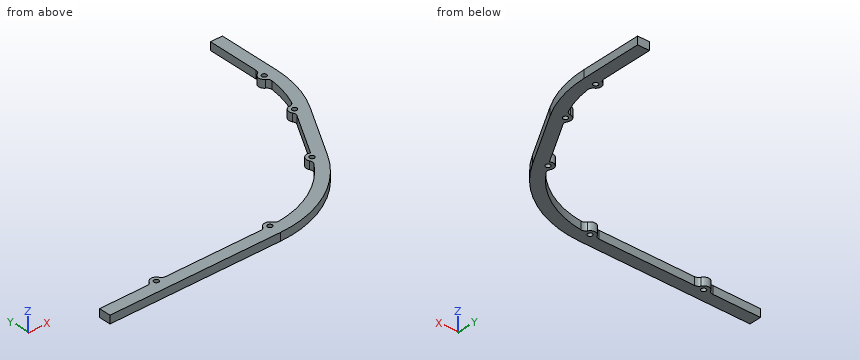
Solid Edge part; units mm, degrees
sketch "Sketch1" plane through (0.0007, 14.651, 5) normal (0, 0, 1) x (1, 0, 0)
  line L0 (-114.0407, 98.8093) -> (-57.2599, 131.5929)
  arc A0 (-54.1474, 131.5247) -> (-57.2599, 131.5929) centre (-55.7598, 128.9948) ccw
  arc A1 (-47.0142, 137.1861) -> (-48.7662, 134.4664) centre (-45.7662, 134.458) ccw
  arc A2 (-47.0142, 137.1861) -> (-26.9146, 142.5706) centre (-21.0226, 80.3698) cw
  arc A3 (-24.0376, 141.0909) -> (-26.9146, 142.5706) centre (-26.6317, 139.5839) ccw
  arc A4 (-15.245, 142.849) -> (-17.9063, 141.2336) centre (-15.245, 139.849) ccw
  line L1 (-15.245, 142.849) -> (15.2436, 142.849)
  arc A5 (17.905, 141.2336) -> (15.2436, 142.849) centre (15.2436, 139.849) ccw
  arc A6 (26.9132, 142.5696) -> (24.036, 141.0904) centre (26.6298, 139.583) ccw
  arc A7 (26.9132, 142.5696) -> (47.0027, 137.1869) centre (21.0099, 80.3561) cw
  arc A8 (48.7549, 134.4673) -> (47.0027, 137.1869) centre (45.7549, 134.4587) ccw
  arc A9 (57.2487, 131.5943) -> (54.1362, 131.526) centre (55.7487, 128.9962) ccw
  line L2 (57.2487, 131.5943) -> (114.0299, 98.8129)
  arc A10 (115.5271, 96.0833) -> (114.0299, 98.8129) centre (112.5299, 96.2148) ccw
  arc A11 (124.0003, 92.7805) -> (120.7849, 92.9052) centre (122.2944, 90.3127) ccw
  arc A12 (124.0003, 92.7805) -> (155.0355, 39.027) centre (82.7747, 33.1424) cw
  arc A13 (153.5358, 36.1799) -> (155.0355, 39.027) centre (152.0454, 38.7835) ccw
  arc A14 (155.2747, 27.3761) -> (153.6593, 30.0375) centre (152.2747, 27.3761) ccw
  line L3 (155.2747, 27.3761) -> (155.2747, -38.192)
  arc A15 (153.6593, -40.8534) -> (155.2747, -38.192) centre (152.2747, -38.192) ccw
  arc A16 (154.9954, -49.8615) -> (153.5161, -46.9844) centre (152.0088, -49.5782) ccw
  arc A17 (154.9954, -49.8615) -> (149.6134, -69.9554) centre (92.7533, -43.9583) cw
  arc A18 (146.8942, -71.7079) -> (149.6134, -69.9554) centre (146.8851, -68.7079) ccw
  arc A19 (144.0217, -80.2016) -> (143.9534, -77.0892) centre (141.4236, -78.7016) ccw
  line L4 (144.0217, -80.2016) -> (127.6444, -108.5679)
  arc A20 (122.7007, -116.5716) -> (122.8583, -113.3403) centre (120.256, -114.8329) ccw
  arc A21 (77.6703, -142.5696) -> (122.7007, -116.5716) centre (71.767, -80.3476) ccw
  arc A22 (74.7931, -141.0904) -> (77.6703, -142.5696) centre (77.3869, -139.583) ccw
  arc A23 (66.0007, -142.849) -> (68.6621, -141.2336) centre (66.0007, -139.849) ccw
  line L5 (5.7656, -142.849) -> (66.0007, -142.849)
  arc A24 (3.1042, -141.2336) -> (5.7656, -142.849) centre (5.7656, -139.849) ccw
  arc A25 (-5.767, -142.849) -> (-3.1056, -141.2336) centre (-5.767, -139.849) ccw
  line L6 (-66.0021, -142.849) -> (-5.767, -142.849)
  arc A26 (-68.6634, -141.2336) -> (-66.0021, -142.849) centre (-66.0021, -139.849) ccw
  arc A27 (-77.6716, -142.5694) -> (-74.7944, -141.0903) centre (-77.3881, -139.5828) ccw
  arc A28 (-122.6994, -116.5717) -> (-77.6716, -142.5694) centre (-71.7665, -80.349) ccw
  arc A29 (-122.857, -113.3404) -> (-122.6994, -116.5717) centre (-120.2547, -114.833) ccw
  arc A30 (-128.7762, -106.6053) -> (-126.0465, -108.1024) centre (-126.1781, -105.1053) ccw
  line L7 (-144.0218, -80.199) -> (-128.7762, -106.6053)
  arc A31 (-143.9535, -77.0865) -> (-144.0218, -80.199) centre (-141.4237, -78.699) ccw
  arc A32 (-149.6144, -69.9531) -> (-146.8949, -71.7053) centre (-146.8862, -68.7053) ccw
  arc A33 (-154.9987, -49.8585) -> (-149.6144, -69.9531) centre (-92.7672, -43.9523) ccw
  arc A34 (-153.5196, -46.9813) -> (-154.9987, -49.8585) centre (-152.0122, -49.5751) ccw
  arc A35 (-155.2786, -38.189) -> (-153.6631, -40.8503) centre (-152.2786, -38.1889) ccw
  line L8 (-155.2818, 27.3758) -> (-155.2786, -38.189)
  arc A36 (-153.6665, 30.0373) -> (-155.2818, 27.3758) centre (-152.2818, 27.376) ccw
  arc A37 (-155.0428, 39.0267) -> (-153.5432, 36.1796) centre (-152.0527, 38.7832) ccw
  arc A38 (-124.0109, 92.7765) -> (-155.0428, 39.0267) centre (-82.7847, 33.1421) ccw
  arc A39 (-120.7955, 92.9014) -> (-124.0109, 92.7765) centre (-122.3049, 90.3088) ccw
  arc A40 (-114.0407, 98.8093) -> (-115.5378, 96.0796) centre (-112.5406, 96.2112) ccw
  arc A41 (-48.7662, 134.4664) -> (-54.1474, 131.5247) centre (-52.2662, 134.4761) cw
  arc A42 (-17.9064, 141.2336) -> (-24.0377, 141.0909) centre (-21.0113, 142.849) cw
  arc A43 (24.036, 141.0904) -> (17.905, 141.2336) centre (21.0099, 142.849) cw
  arc A44 (54.1362, 131.526) -> (48.7549, 134.4673) centre (52.2549, 134.4774) cw
  arc A45 (120.7849, 92.9052) -> (115.5271, 96.0832) centre (119.0237, 95.9298) cw
  arc A46 (153.6593, 30.0375) -> (153.5358, 36.1799) centre (155.2747, 33.1424) cw
  arc A47 (153.5161, -46.9844) -> (153.6593, -40.8534) centre (155.2747, -43.9583) cw
  arc A48 (143.9534, -77.0891) -> (146.8942, -71.7079) centre (146.9048, -75.2079) cw
  arc A49 (122.8584, -113.3404) -> (127.6444, -108.5679) centre (125.8944, -111.599) cw
  arc A50 (68.6621, -141.2336) -> (74.7931, -141.0904) centre (71.767, -142.849) cw
  arc A51 (-3.1056, -141.2336) -> (3.1042, -141.2336) centre (-0.0007, -142.849) cw
  arc A52 (-74.7944, -141.0903) -> (-68.6635, -141.2336) centre (-71.7684, -142.849) cw
  arc A53 (-126.0466, -108.1024) -> (-122.857, -113.3404) centre (-125.8931, -111.599) cw
  arc A54 (-146.8949, -71.7053) -> (-143.9536, -77.0866) centre (-146.905, -75.2053) cw
  arc A55 (-153.6632, -40.8503) -> (-153.5196, -46.9813) centre (-155.2784, -43.9553) cw
  arc A56 (-153.5432, 36.1796) -> (-153.6665, 30.0373) centre (-155.2821, 33.1421) cw
  arc A57 (-115.5377, 96.0796) -> (-120.7955, 92.9014) centre (-119.0344, 95.926) cw
  line L9 (-56.0166, 140.971) -> (-122.7845, 102.4212)
  arc A58 (-162.7821, 33.1421) -> (-122.7845, 102.4212) centre (-82.7847, 33.1421) cw
  line L10 (-162.7821, 33.1421) -> (-162.7784, -43.9553)
  arc A59 (-162.7784, -43.9553) -> (-153.4002, -78.9553) centre (-92.7784, -43.9553) ccw
  line L11 (-132.3882, -115.349) -> (-153.4002, -78.9553)
  arc A60 (-132.3882, -115.349) -> (-71.7683, -150.349) centre (-71.7665, -80.349) ccw
  line L12 (71.767, -150.349) -> (-71.7683, -150.349)
  arc A61 (71.767, -150.349) -> (132.3896, -115.349) centre (71.7678, -80.349) ccw
  line L13 (132.3896, -115.349) -> (153.4002, -78.9576)
  arc A62 (162.7747, -43.9583) -> (153.4002, -78.9576) centre (92.791, -43.9684) cw
  line L14 (162.7747, 33.1424) -> (162.7747, -43.9583)
  arc A63 (122.7736, 102.4251) -> (162.7747, 33.1424) centre (82.7747, 33.1424) cw
  line L15 (56.0045, 140.9728) -> (122.7736, 102.4251)
  arc A64 (21.0099, 150.349) -> (56.0045, 140.9728) centre (21.008, 80.349) cw
  line L16 (-21.0112, 150.349) -> (21.0099, 150.349)
  arc A65 (-32.5074, 149.4015) -> (-21.0112, 150.349) centre (-20.997, 79.961) cw
  arc A66 (-44.641, 146.2432) -> (-32.5074, 149.4015) centre (-21.0122, 80.3518) cw
  arc A67 (-56.0166, 140.971) -> (-44.641, 146.2432) centre (-21.0122, 80.3518) cw
  circle A68 centre (-71.7683, -142.849) radius 1.5
  circle A69 centre (-0.0007, -142.849) radius 1.5
  circle A70 centre (-125.893, -111.599) radius 1.5
  circle A71 centre (-146.905, -75.2053) radius 1.5
  circle A72 centre (-155.2784, -43.9553) radius 1.5
  circle A73 centre (-155.2821, 33.1421) radius 1.5
  circle A74 centre (-119.0344, 95.9261) radius 1.5
  circle A75 centre (-52.2662, 134.4761) radius 1.5
  circle A76 centre (-21.0112, 142.849) radius 1.5
  circle A77 centre (21.0099, 142.849) radius 1.5
  circle A78 centre (52.2549, 134.4774) radius 1.5
  circle A79 centre (119.0237, 95.9298) radius 1.5
  circle A80 centre (155.2747, 33.1424) radius 1.5
  circle A81 centre (155.2747, -43.9583) radius 1.5
  circle A82 centre (146.9048, -75.2079) radius 1.5
  circle A83 centre (125.8944, -111.599) radius 1.5
  circle A84 centre (71.767, -142.849) radius 1.5
extrude "ExtrudedProtrusion_7" add sketch "Sketch1" along normal blind 5
sketch "Sketch2" plane through (-0.003, 14.651, 10) normal (0, 0, 1) x (1, 0, 0)
  line L0 (-168.1883, -5.4066) -> (170.0115, -5.4066)
  line L1 (170.0115, -5.4066) -> (170.0115, 153.6029)
  line L2 (170.0115, 153.6029) -> (-168.1883, 153.6029)
  line L3 (-168.1883, 153.6029) -> (-168.1883, -5.4066)
extrude "Cutout1" cut sketch "Sketch2" against normal up to next
sketch "Sketch3" plane through (-0.0021, -63.2268, 10) normal (0, 0, 1) x (1, 0, 0)
  line L0 (-35.8817, -72.4712) -> (-192.1854, -72.4712)
  line L1 (-192.1854, -72.4712) -> (-192.1854, 77.1316)
  line L2 (-192.1854, 77.1316) -> (-35.8817, 77.1316)
  line L3 (-35.8817, 77.1316) -> (-35.8817, -72.4712)
extrude "Cutout2" cut sketch "Sketch3" against normal up to next
properties material "Polycarbonate"
Design review of the part built by this model. Coordinates are the model's own, in mm. Round coordinates to 2 decimals unless told otherwise and drop trailing zeros. Write each loop counter-clockwise with the first axis right and the second up, starting at its lowest first coordinate (ties: lowest second). Pieces come first, ordered by that corner, then holes.
Item 1: For pin 1 Ø2.5 at (x, z) = (-23, 6.5) entering from +Y; pin 2 Ø1.5 at (y, z) = (-0.5, 6.5) entering from -X; pin 3 Ø1 at (x, z) = (69, 8) entering from +Y, all flat-tipped, find the tip position at first contact; note any pin that passes through.
Item 2: Consider section A-A on z = 8.8. Count the separate pieces of the cut face and the enclosed holes in it, and give its area (3 significant figures).
Item 3: Wall thickness on L1, parallel to Y at x = 10, z = 9; L2, parallel to X at y = -12.5, z = 6.4; L3, parallel to Y at x = 4.5, z = 5.65: over which ranges is each line inside the solid? List them lowest first.
Item 4: Consider section C-C on y = -121.5. Give the boundary of the cut face in (x, z).
Item 5: Consider section B-B on x = -11.5. Give the boundary of the cut face in (y, z), and give its area (3 significant figures).
Check values:
1. pin 1: stops at y = -128.2
1. pin 2: stops at x = 155.28
1. pin 3: stops at y = -125.53
2. separate pieces: 1
2. enclosed holes: 5
2. area: 2,260 mm2
3. L1: y = -135.7 to -128.2
3. L2: x = 155.28 to 162.78
3. L3: y = -135.7 to -127.92
4. outline: (99.92, 5) - (114.03, 5) - (114.03, 10) - (99.92, 10) - close
5. outline: (-135.7, 5) - (-128.2, 5) - (-128.2, 10) - (-135.7, 10) - close
5. area: 37.5 mm2
